Could you check a few things on this drawing? It's one solid part, dimensions in mm from its lowest x, y, z. A direction names the side the tool comes from. Round coordinates to 2 decimals unless told otherwise and drop trailing zeros. Loops run counter-clockwise (first coordinate to the right, second up) from the corner with the lowest first, then second, coordinate; pieces in that order, holes last. Notation, with made-up numbers: M 73,59.25 L 92,59.25 A14 ccw 92,67.25 Z; hole C 37.5,27.5 d4. An arc over 180 degrees is marked long. Write item = value, one per line. Start each with the question number.
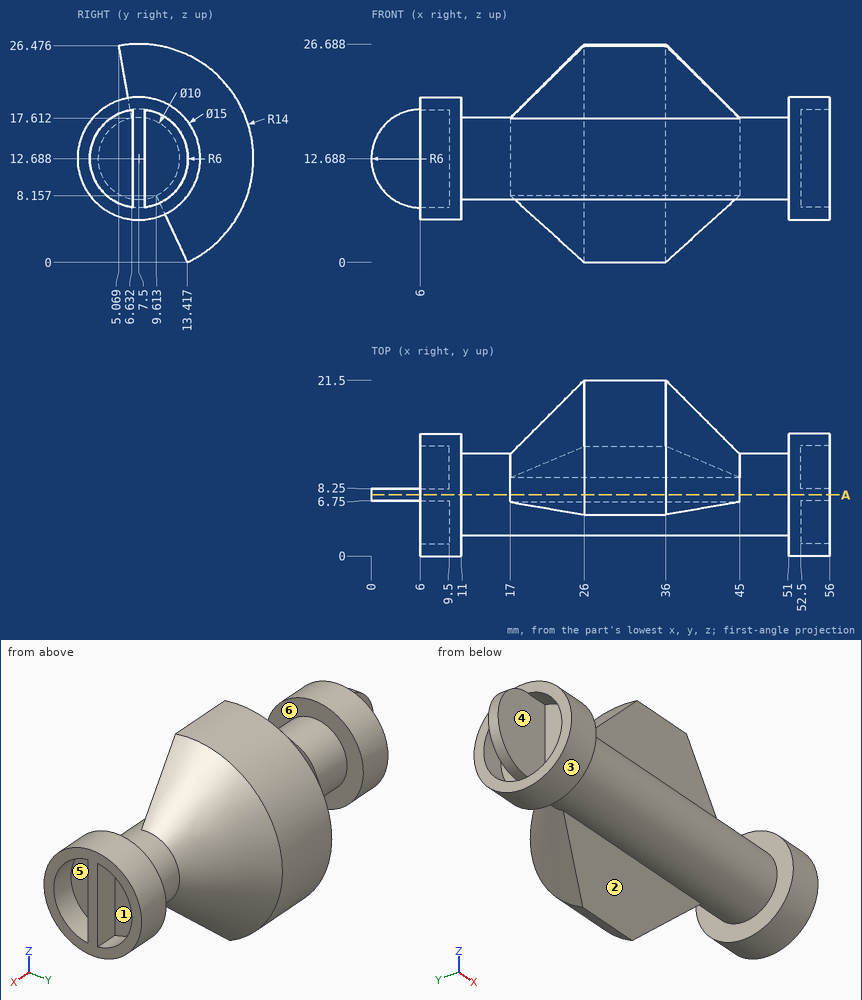
Item 1: We'd pull the mould along X, two halves only. Please class the marked faces 1, 2 and 3: released by +X, released by -X, zero draft, split by the parting line, or undercut.
Item 2: Will these pins go through, and if not, where does the flat tip stop? pin 1 Ø1 at (x, y) = (8.5, 11.5) entering from +Z; pin 2 Ø5 at (x, y) = (28, 11) entering from +Z; pin 3 Ø2.5 at (y, z) = (10.5, 9.5) entering from -X; pin 4 Ø7.5 at (y, z) = (8, 10.5) entering from -X.
Item 3: I want a section at A-A, the plane y = 7.5. List the corners of the cut face in (x, z) for me.
Item 4: Please list where these lines run through material, in increasing order: line 1 (X direction, y = 5, z = 19.5); line 2 (X direction, y = 11.25, z = 10); line 3 (X direction, y = 17, z = 17.75) (1 decimal). Write a range as [from, to].
Item 5: For the marked faces 4, 5 and 6, which set-ups out of +Z, -Z, +X, -X, +Y, -Y let a thin tool reach every point of the face, with its end or its side?
Worked out:
q1.face_1 = released by +X
q1.face_2 = undercut
q1.face_3 = zero draft
q2.pin_1 = 19.32
q2.pin_2 = 26.65
q2.pin_3 = 9.5
q2.pin_4 = 0
q3.outline = M 6,5.19 L 11,5.19 L 11,7.69 L 51,7.69 L 51,5.19 L 56,5.19 L 56,20.19 L 51,20.19 L 51,17.69 L 45,17.69 L 36,26.69 L 26,26.69 L 17,17.69 L 11,17.69 L 11,20.19 L 6,20.19 L 6,18.69 A6 ccw 6,6.69 Z
q4.line_1 = [6, 11], [51, 56]
q4.line_2 = [9.5, 52.5]
q4.line_3 = [22.8, 39.2]
q5.face_4 = -X
q5.face_5 = +X
q5.face_6 = none
